The listing builds one solid part. Answer for the finished solid, in the listing's coordinates (mm). A direction names the side the tool comes from. Round coordinates to 2 decimals unless told otherwise and drop trailing zeros. Loops run counter-clockwise (first coordinate to the right, second up) from the corner with the lowest first, then second, coordinate; pieces in that order, holes last. Notation, with made-up numbers: M -6.75,46.5 L 45.25,46.5 A14 cw 45.25,63.5 Z; hole C 35.25,50.25 d8. An arc over 180 degrees is marked long. Put each result on its own line as item: value. Start each with the question number.
(1) Which of the six approach directions +Z, -Z, +X, -X, +Y, -Y give full straight-line access (tool end or side, diameter ignored) to faces 4 (the face through (-3.234, 10.037, 2.48)), 5 (the face through (-1.5, 6.46, 0.07)), 6 (the face through (-4, 17.1, -2))?
(2) Section C-C, the plane y = 5.25 is taken. Determine the outline of the cut face in (x, z), then the cut area to 3 significant figures.
(3) Flat-ended cylindrical pins translate along their axes: P1, Ø3, axis at x = 0, z = 0.5, coming from the +Y side; P2, Ø5, axis at x = -4, y = 7, coming from the -Z side; P3, Ø6, axis at y = 4.5, z = -1.5, coming from the +X side. Find the tip coordinate at first contact, or state that the pin passes through.
(4) Section B-B, the plane y = 1.5 is taken. Determine the outline of the cut face in (x, z), then the cut area to 3 significant figures.
(5) Straight lines are drawn through the part: line 1 (Z direction, x = 0, y = 18); line 2 (X direction, y = 16, z = 0). For each, find the intervals that lie inside material, in ascending order.
(6) Determine the mould class of faces 1 (the face through (-4, 11, -2)), 2 (the face through (1.3, 13.1, 1.3)), 3 (the face through (-1.19, 14.02, 5.37)) for opening direction X: released by +X, released by -X, zero draft, split by the parting line, or undercut.
```python
from build123d import *

# Parameters (mm, degrees)
SKETCH1_R           = 3.15
BOSS_EXTRUDE1_DEPTH = 8.5
BOSS_EXTRUDE1_TAPER = -1.35
SKETCH2_R           = 4.075
BOSS_EXTRUDE2_DEPTH = 2.5
SKETCH3_R           = 5.5
BOSS_EXTRUDE3_DEPTH = 6.1
SKETCH4_R           = 4.25
BOSS_EXTRUDE4_DEPTH = 2.5
SKETCH5_R           = 3
CUT_EXTRUDE1_DEPTH  = 6.5
SKETCH6_R           = 1.5
CUT_EXTRUDE2_DEPTH  = 13.1
FILLET1_R           = 0.6


with BuildPart() as part:
    # Sketch1 → Boss-Extrude1 (new body)
    with BuildSketch(Plane(origin=(0, 0, 0), x_dir=(1, 0, 0), z_dir=(0, 1, 0))):
        Circle(SKETCH1_R)
    extrude(amount=BOSS_EXTRUDE1_DEPTH, taper=BOSS_EXTRUDE1_TAPER)

    # Sketch2 → Boss-Extrude2 (add)
    with BuildSketch(Plane(origin=(0, 8.5, 0), x_dir=(1, 0, 0), z_dir=(0, 1, 0))):
        Circle(SKETCH2_R)
    extrude(amount=BOSS_EXTRUDE2_DEPTH)

    # Sketch3 → Boss-Extrude3 (add)
    with BuildSketch(Plane(origin=(0, 11, 0), x_dir=(1, 0, 0), z_dir=(0, 1, 0))):
        Circle(SKETCH3_R)
    extrude(amount=BOSS_EXTRUDE3_DEPTH)

    # Sketch4 → Boss-Extrude4 (add)
    with BuildSketch(Plane(origin=(0, 17.1, 0), x_dir=(1, 0, 0), z_dir=(0, 1, 0))):
        Circle(SKETCH4_R)
    extrude(amount=BOSS_EXTRUDE4_DEPTH)

    # Sketch5 → Cut-Extrude1 (cut)
    with BuildSketch(Plane(origin=(0, 19.6, 0), x_dir=(1, 0, 0), z_dir=(0, 1, 0))):
        Circle(SKETCH5_R)
    extrude(amount=-CUT_EXTRUDE1_DEPTH, mode=Mode.SUBTRACT)

    # Sketch6 → Cut-Extrude2 (cut)
    with BuildSketch(Plane.XZ):
        Circle(SKETCH6_R)
    extrude(amount=-CUT_EXTRUDE2_DEPTH, mode=Mode.SUBTRACT)

    # Fillet1
    fillet1_edges = [part.edges().sort_by_distance(p)[0] for p in [
        (-5.5, 17.1, 0),
        (-4.25, 19.6, 0),
        (-4.075, 8.5, 0),
        (-5.5, 11, 0),
    ]]
    fillet(fillet1_edges, radius=FILLET1_R)


solid = part.part
```
Recorded:
1. face 4: -Y
1. face 5: +Y, -Y
1. face 6: +Y
2. outline: C 0,0 d6.55; hole C 0,0 d3
2. area: 26.6 mm²
3. P1: stops at y = 13.1
3. P2: stops at z = -3.29
3. P3: stops at x = 3.32
4. outline: C 0,0 d6.37; hole C 0,0 d3
4. area: 24.8 mm²
5. line 1: z = -4.25 to -3, 3 to 4.25
5. line 2: x = -5.5 to -3, 3 to 5.5
6. face 1: zero draft
6. face 2: undercut
6. face 3: split by the parting line
